Here's how the part is built. I have some questions about the finished solid (model axes, mm). A direction names the side the tool comes from. Give positions to 0.01 mm unless a question says otherwise; leave off trailing zeros. Order: outer loops, then holes, each group sorted by start corner. A loop starts at its lowest first (then second) coordinate and runs counter-clockwise, first axis right, second up.
from build123d import *

# Parameters (mm, degrees)
SKETCH1_R                 = 1.651
BOSS_EXTRUDE2_DEPTH       = 5.3975
SKETCH2_R                 = 1.143
CUT_EXTRUDE1_DEPTH        = 6.3975
SKETCH3_R                 = 12.1285
CUT_EXTRUDE2_DEPTH        = 6.3975
SKETCH4_W                 = 28.562713242
SKETCH4_H                 = 11.677503754
BOSS_EXTRUDE3_DEPTH       = 5.3975
SKETCH5_W                 = 230.699333954
SKETCH5_H                 = 107.587024537
CUT_EXTRUDE3_DEPTH        = 6.3975
CUT_EXTRUDE4_DEPTH        = 6.3975
SKETCH156_W               = 11.43
SKETCH156_H               = 10.16
CUT_EXTRUDE152_DEPTH      = 6.3975
SKETCH164_R               = 1.651
CUT_EXTRUDE160_DEPTH      = 21.59
SKETCH218_R               = 3.175
CUT_EXTRUDE214_DEPTH      = 103.378
CUT_EXTRUDE214_DEPTH_BACK = 48.768
CUT_EXTRUDE155_DEPTH      = 34.544
FILLET1_R                 = 2.54


with BuildPart() as part:
    # Sketch1 → Boss-Extrude2 (new body)
    with BuildSketch(Plane.XY):
        with BuildLine():
            Line((-65.2537815, 36.83), (-54.8397815, 36.83))
            Line((-54.8397815, 36.83), (-54.8397815, -36.83))
            Line((-54.8397815, -36.83), (-65.2537815, -36.83))
            ThreePointArc((-65.2537815, -36.83), (0, -74.93), (65.2537815, -36.83))
            Line((65.2537815, -36.83), (54.8397815, -36.83))
            Line((54.8397815, -36.83), (54.8397815, 36.83))
            Line((54.8397815, 36.83), (65.2537815, 36.83))
            ThreePointArc((65.2537815, 36.83), (0, 74.93), (-65.2537815, 36.83))
        make_face()
        with Locations((-45.466, 11.049)):
            Circle(SKETCH1_R, mode=Mode.SUBTRACT)
        with Locations((-20.067270032, 10.795)):
            Circle(SKETCH1_R, mode=Mode.SUBTRACT)
        with Locations((-20.067270032, -10.795)):
            Circle(SKETCH1_R, mode=Mode.SUBTRACT)
        with Locations((-45.466, -11.049)):
            Circle(SKETCH1_R, mode=Mode.SUBTRACT)
        with Locations((45.466, -11.049)):
            Circle(SKETCH1_R, mode=Mode.SUBTRACT)
        with Locations((20.067270032, -10.795)):
            Circle(SKETCH1_R, mode=Mode.SUBTRACT)
        with Locations((20.067270032, 10.795)):
            Circle(SKETCH1_R, mode=Mode.SUBTRACT)
        with Locations((45.466, 11.049)):
            Circle(SKETCH1_R, mode=Mode.SUBTRACT)
    extrude(amount=BOSS_EXTRUDE2_DEPTH)

    # Sketch2 → Cut-Extrude1 (cut, through all)
    with BuildSketch(Plane.XY.offset(5.3975)):
        with Locations((-6.731, 62.23)):
            Circle(SKETCH2_R)
        with Locations((6.731, 62.23)):
            Circle(SKETCH2_R)
    extrude(amount=-CUT_EXTRUDE1_DEPTH, mode=Mode.SUBTRACT)

    # Sketch3 → Cut-Extrude2 (cut, through all)
    with BuildSketch(Plane(origin=(0, 0, 0), x_dir=(-1, 0, 0), z_dir=(0, 0, -1))):
        with Locations((-42.926, -42.926)):
            Circle(SKETCH3_R)
        with Locations((14.224, -34.29)):
            Circle(SKETCH3_R)
        with Locations((14.224, 34.29)):
            Circle(SKETCH3_R)
        with Locations((-42.926, 42.926)):
            Circle(SKETCH3_R)
        with Locations((42.926, 42.926)):
            Circle(SKETCH3_R)
        with Locations((-14.224, 34.29)):
            Circle(SKETCH3_R)
        with Locations((-14.224, -34.29)):
            Circle(SKETCH3_R)
        with Locations((42.926, -42.926)):
            Circle(SKETCH3_R)
    extrude(amount=-CUT_EXTRUDE2_DEPTH, mode=Mode.SUBTRACT)

    # Sketch4 → Boss-Extrude3 (add)
    with BuildSketch(Plane(origin=(0, 0, 0), x_dir=(-1, 0, 0), z_dir=(0, 0, -1))):
        with Locations((-1.488809975, 62.152540216)):
            Rectangle(SKETCH4_W, SKETCH4_H)
    extrude(amount=-BOSS_EXTRUDE3_DEPTH)

    # Sketch5 → Cut-Extrude3 (cut, through all)
    with BuildSketch(Plane(origin=(0, 0, 0), x_dir=(-1, 0, 0), z_dir=(0, 0, -1))):
        with Locations((1.971047261, -36.648512269)):
            Rectangle(SKETCH5_W, SKETCH5_H)
    extrude(amount=-CUT_EXTRUDE3_DEPTH, mode=Mode.SUBTRACT)

    # Sketch6 → Cut-Extrude4 (cut, through all)
    with BuildSketch(Plane(origin=(0, 0, 0), x_dir=(-1, 0, 0), z_dir=(0, 0, -1))):
        Polygon((4.498, 63.592546635), (6.858, 64.955093271), (9.218, 63.592546635), (9.218, 60.867453365), (6.858, 59.504906729), (4.498, 60.867453365), align=None)
        Polygon((-6.858, 64.955093271), (-9.218, 63.592546635), (-9.218, 60.867453365), (-6.858, 59.504906729), (-4.498, 60.867453365), (-4.498, 63.592546635), align=None)
    extrude(amount=-CUT_EXTRUDE4_DEPTH, mode=Mode.SUBTRACT)

    # Sketch156 → Cut-Extrude152 (cut, through all)
    with BuildSketch(Plane(origin=(0, 0, 0), x_dir=(-1, 0, 0), z_dir=(0, 0, -1))):
        with Locations((33.8847815, 22.225)):
            Rectangle(SKETCH156_W, SKETCH156_H)
        with Locations((-33.8847815, 22.225)):
            Rectangle(SKETCH156_W, SKETCH156_H)
    extrude(amount=-CUT_EXTRUDE152_DEPTH, mode=Mode.SUBTRACT)

    # Sketch164 → Cut-Extrude160 (cut)
    with BuildSketch(Plane(origin=(0, 0, 0), x_dir=(-1, 0, 0), z_dir=(0, 0, -1))):
        with Locations((25.8572, 45.466)):
            Circle(SKETCH164_R)
        with Locations((-25.8572, 45.466)):
            Circle(SKETCH164_R)
    extrude(amount=-CUT_EXTRUDE160_DEPTH, mode=Mode.SUBTRACT)

    # Sketch218 → Cut-Extrude214 (cut, two sides)
    with BuildSketch(Plane(origin=(30.092005081, 4.08352975, 11.4935), x_dir=(-1, 0, 0), z_dir=(0, 0, -1))) as cut_extrude214_sk:
        with Locations((-16.897994919, 21.31647025)):
            Circle(SKETCH218_R)
        with Locations((77.082005081, 21.31647025)):
            Circle(SKETCH218_R)
        with Locations((30.092005081, 21.31647025)):
            Circle(SKETCH218_R)
    extrude(amount=CUT_EXTRUDE214_DEPTH, mode=Mode.SUBTRACT)
    extrude(cut_extrude214_sk.sketch, amount=-CUT_EXTRUDE214_DEPTH_BACK, mode=Mode.SUBTRACT)

    # Sketch159 → Cut-Extrude155 (cut)
    with BuildSketch(Plane(origin=(0, 0, 0), x_dir=(-1, 0, 0), z_dir=(0, 0, -1))):
        with BuildLine():
            Line((-12.7, 20.24), (-8.888991966, 20.24))
            ThreePointArc((-8.888991966, 20.24), (-5.715, 23.495), (-2.541008034, 20.24))
            Line((-2.541008034, 20.24), (2.541008034, 20.24))
            ThreePointArc((2.541008034, 20.24), (5.715, 23.495), (8.888991966, 20.24))
            Line((8.888991966, 20.24), (12.7, 20.24))
            ThreePointArc((12.7, 20.24), (17.7, 15.24), (12.7, 10.24))
            Line((12.7, 10.24), (-12.7, 10.24))
            ThreePointArc((-12.7, 10.24), (-17.7, 15.24), (-12.7, 20.24))
        make_face()
    extrude(amount=-CUT_EXTRUDE155_DEPTH, mode=Mode.SUBTRACT)

    # Fillet1
    fillet1_edges = [part.edges().sort_by_distance(p)[0] for p in [
        (-39.5997815, 17.145, 2.69875),
        (-28.1697815, 17.145, 2.69875),
        (28.1697815, 17.145, 2.69875),
        (39.5997815, 17.145, 2.69875),
        (17.322875188, 17.145, 2.69875),
        (-17.322875188, 17.145, 2.69875),
        (8.888991966, 20.24, 2.69875),
        (2.541008034, 20.24, 2.69875),
        (-2.541008034, 20.24, 2.69875),
        (-8.888991966, 20.24, 2.69875),
    ]]
    fillet(fillet1_edges, radius=FILLET1_R)


solid = part.part
Q1. If we section it at D-D on x = -46.99: List the corners of the cut face in (y, z) for me (1 decimal).
Filled sheet:
outline: (17.1, 0) - (22.2, 0) - (22.2, 5.4) - (17.1, 5.4) - close; (28.6, 0) - (31.5, 0) - (31.5, 5.4) - (28.6, 5.4) - close; (54.4, 0) - (58.4, 0) - (58.4, 5.4) - (54.4, 5.4) - close
Q2. Thinking about a two-plate mould opening in Y: for faces 6 (the face through (-9.218, 62, 3)), 7 (the face through (34, 27.305, 3)), 8 (the face through (1.11, 74.92, 2.66)), which applies, released by +Y, released by -Y, zero draft, split by the parting line, or undercut?
Filled sheet:
face 6: undercut
face 7: released by -Y
face 8: released by +Y
Q3. I'm going to push flat-ended pins straight in: P1, Ø3, axis at x = -48.5, z = 2, coming from the +Y side; P2, Ø2.5, axis at y = 24, z = 2, coming from the +X side; P3, Ø1.6, axis at x = 31.5, z = 2.5, coming from the -Y side (3 decimals); P4, Ø14.5, axis at x = 42.926, y = 42.926, coming from the -Z side. Where does each tip first touch, or does it pass through?
Filled sheet:
P1: stops at y = 58.36
P2: stops at x = 54.84
P3: stops at y = 27.305
P4: passes through
Q4. If we section it at B-B on y = 34.29: List the corners of the cut face in (x, z) for me, plus the area to 3 significant figures.
Filled sheet:
outline: (-54.84, 0) - (-51.44, 0) - (-51.44, 5.4) - (-54.84, 5.4) - close; (-34.41, 0) - (-26.35, 0) - (-26.35, 5.4) - (-34.41, 5.4) - close; (-2.1, 0) - (2.1, 0) - (2.1, 5.4) - (-2.1, 5.4) - close; (26.35, 0) - (34.41, 0) - (34.41, 5.4) - (26.35, 5.4) - close; (51.44, 0) - (54.84, 0) - (54.84, 5.4) - (51.44, 5.4) - close
area: 146 mm2
Q5. If we section it at A-A on x = 47.5: List the corners of the cut face in (y, z) for me (1 decimal).
Filled sheet:
outline: (17.1, 0) - (22.3, 0) - (22.3, 5.4) - (17.1, 5.4) - close; (28.5, 0) - (31.7, 0) - (31.7, 5.4) - (28.5, 5.4) - close; (54.2, 0) - (58, 0) - (58, 5.4) - (54.2, 5.4) - close
Q6. For faces 1 (the face through (-4.498, 62, 3)), 2 (the face through (-48, 17.145, 3)), 3 (the face through (-54.84, 27, 3)), 4 (the face through (-39.6, 23, 3)), 5 (the face through (60, 36.83, 3)), which set-ups out of +Z, -Z, +X, -X, +Y, -Y let a thin tool reach every point of the face, with its end or its side?
Filled sheet:
face 1: +Z, -Z
face 2: +Z, -Z, +X, -X, -Y
face 3: +Z, -Z, -X, -Y
face 4: +Z, -Z, -Y
face 5: +Z, -Z, +X, -Y
Q7. If we section it at C-C on x = 34: List the corners of the cut face in (y, z) for me (1 decimal), plus the area to 3 significant figures.
Filled sheet:
outline: (27.3, 0) - (34.7, 0) - (34.7, 5.4) - (27.3, 5.4) - close; (51.1, 0) - (66.8, 0) - (66.8, 5.4) - (51.1, 5.4) - close
area: 124 mm2
Q8. I need wall thicknesses on L1, parallel to X at y = 37, z = 5; L2, parallel to Y at x = 46.99, z = 3.1 (3 decimals); L3, parallel to Y at x = 0, z = 1.1 (3 decimals). Which ranges of each line are inside material? Lowest first, please.
Filled sheet:
L1: x = -65.16 to -53.51, -32.34 to -26.05, -2.4 to 2.4, 26.05 to 32.34, 53.51 to 65.16
L2: y = 17.145 to 22.225, 28.575 to 31.499, 54.353 to 58.365
L3: y = 20.24 to 22.225, 28.575 to 74.93
